Can you work these out from the model? Positions are in its coordinate system, mm. Coordinates: 2 decimals unless noted, no trailing zeros. Order: outer loops, then holes, each group sorted by start corner. A loop starts at its lowest first (then second) coordinate and runs counter-clockwise, first axis right, second up. Notation, with made-up numbers: (41, 46) - (73, 46) arc R13 cw to (73, 65) - close; hole circle Ø5 at (44, 22.25). An arc over 180 degrees is marked (long way). Return JSON: item names as keys, results as strings. Group by question number.
1) For pin 1 Ø0.8 at (y, z) = (-25.5, 1.5) entering from +X; pin 2 Ø1.2 at (y, z) = (97.5, 1.5) entering from -X; pin 3 Ø1.2 at (x, z) = (-18, 1) entering from -Y, each with a flat end and sliding along its axis, tell me the tip position at first contact or that it passes through.
2) Imagine slicing it at A-A (y = 120). Write out the boundary of the cut face in (x, z).
3) Imagine slicing it at D-D (x = -31.9). Write out the boundary of the cut face in (y, z), and give its area (3 significant figures).
4) If I drill on line 1 along Y through (x, z) = (-12.4, 1.3); line 2 along Y through (x, z) = (44, 1.05); line 3 along Y through (x, z) = (11, 1.35), over which ranges is the centre line in solid material (lowest first)?
5) Imagine slicing it at C-C (x = 2). Write out the boundary of the cut face in (y, z).
6) Imagine slicing it at B-B (x = -12.4). Write out the boundary of the cut face in (y, z).
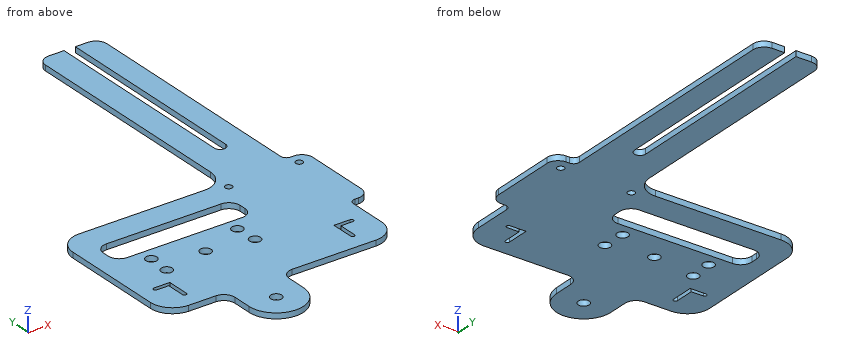
```python
from build123d import *

# Parameters (mm, degrees)
SKETCH1_W           = 200
SKETCH1_H           = 300
SKETCH1_W_2         = 96.214780988
SKETCH1_H_2         = 20
BOSS_EXTRUDE1_DEPTH = 2.5
SKETCH2_R           = 2.5
CUT_EXTRUDE1_DEPTH  = 10
CUT_EXTRUDE3_DEPTH  = 10
CUT_EXTRUDE4_REACH  = 182.936
SKETCH5_W           = 62
SKETCH5_H           = 13
FILLET2_R           = 5
FILLET3_R           = 10
FILLET4_R           = 5
CUT_EXTRUDE6_REACH  = 182.936
SKETCH7_R           = 1.6
FILLET5_R           = 2.5
CUT_EXTRUDE7_REACH  = 182.936
SKETCH8_R           = 2.5


with BuildPart() as part:
    # Sketch1 → Boss-Extrude1 (new body)
    with BuildSketch(Plane.XY):
        Rectangle(SKETCH1_W, SKETCH1_H)
        with Locations((51.892609506, 160)):
            Rectangle(SKETCH1_W_2, SKETCH1_H_2)
    extrude(amount=BOSS_EXTRUDE1_DEPTH)

    # Sketch2 → Cut-Extrude1 (cut)
    with BuildSketch(Plane.XY.offset(2.5)):
        with Locations((-12.4, -28.75)):
            Circle(SKETCH2_R)
        with Locations((7.6, 11.65)):
            Circle(SKETCH2_R)
        with Locations((-32.4, 11.65)):
            Circle(SKETCH2_R)
        Polygon((-44.5, 1.45), (-44.5, 3.25), (-37.2, 3.25), (-37.2, -7.05), (-39, -7.05), (-39, 1.45), align=None)
        Polygon((39, 1.45), (44.5, 1.45), (44.5, 3.25), (37.2, 3.25), (37.2, -7.05), (39, -7.05), align=None)
        with BuildLine():
            Line((-44.5, 1.45), (-44.5, 3.25))
            ThreePointArc((-44.5, 3.25), (-45.4, 2.35), (-44.5, 1.45))
        make_face()
        with BuildLine():
            ThreePointArc((-37.2, -7.05), (-38.1, -7.95), (-39, -7.05))
            Line((-39, -7.05), (-37.2, -7.05))
        make_face()
        with BuildLine():
            ThreePointArc((39, -7.05), (38.1, -7.95), (37.2, -7.05))
            Line((37.2, -7.05), (39, -7.05))
        make_face()
        with BuildLine():
            ThreePointArc((44.5, 3.25), (45.4, 2.35), (44.5, 1.45))
            Line((44.5, 1.45), (44.5, 3.25))
        make_face()
    extrude(amount=-CUT_EXTRUDE1_DEPTH, mode=Mode.SUBTRACT)

    # Sketch4 → Cut-Extrude3 (cut)
    with BuildSketch(Plane.XY.offset(2.5)):
        with BuildLine():
            Line((42.1, 170), (37, 170))
            Line((37, 170), (37, 77))
            ThreePointArc((37, 77), (39.55, 74.45), (42.1, 77))
            Line((42.1, 77), (42.1, 170))
        make_face()
        with BuildLine():
            Line((25, 53), (25, 170))
            Line((25, 170), (3.785219012, 170))
            Line((3.785219012, 170), (3.785219012, 150))
            Line((3.785219012, 150), (-100, 150))
            Line((-100, 150), (-100, -150))
            Line((-100, -150), (100, -150))
            Line((100, -150), (100, 170))
            Line((100, 170), (52.8, 170))
            Line((52.8, 170), (52.8, 55))
            Line((52.8, 55), (61.9, 55))
            Line((61.9, 55), (61.9, 15))
            Line((61.9, 15), (52.8, 15))
            Line((52.8, 15), (52.8, -15))
            Line((52.8, -15), (-0.095794877, -15))
            Line((-0.095794877, -15), (-0.095794877, -28.75))
            ThreePointArc((-0.095794877, -28.75), (-12.4, -41.054205123), (-24.704205123, -28.75))
            Line((-24.704205123, -28.75), (-24.704205123, -15))
            Line((-24.704205123, -15), (-52, -15))
            Line((-52, -15), (-52, 53))
            Line((-52, 53), (25, 53))
        make_face()
    extrude(amount=-CUT_EXTRUDE3_DEPTH, mode=Mode.SUBTRACT)

    # Sketch5 → Cut-Extrude4 (cut, up to next)
    with BuildSketch(Plane.XY.offset(2.5), mode=Mode.PRIVATE) as cut_extrude4_sk1:
        with Locations((-12.4, 34.409289568)):
            Rectangle(SKETCH5_W, SKETCH5_H)
    cut_extrude4_tool1 = extrude(cut_extrude4_sk1.sketch, amount=-CUT_EXTRUDE4_REACH, mode=Mode.PRIVATE) & part.part
    add(cut_extrude4_tool1.solids().sort_by_distance((-12.4, 34.40929, 2.5))[0], mode=Mode.SUBTRACT)

    # Fillet2
    fillet2_edges = [part.edges().sort_by_distance(p)[0] for p in [
        (-43.4, 40.909289568, 1.25),
        (18.6, 40.909289568, 1.25),
        (18.6, 27.909289568, 1.25),
        (-43.4, 27.909289568, 1.25),
    ]]
    fillet(fillet2_edges, radius=FILLET2_R)

    # Fillet3
    fillet3_edges = [part.edges().sort_by_distance(p)[0] for p in [
        (52.8, -15, 1.25),
        (25, 53, 1.25),
        (-52, 53, 1.25),
        (-52, -15, 1.25),
    ]]
    fillet(fillet3_edges, radius=FILLET3_R)

    # Fillet4
    fillet4_edges = [part.edges().sort_by_distance(p)[0] for p in [
        (-0.095794877, -15, 1.25),
        (61.9, 15, 1.25),
        (61.9, 55, 1.25),
        (-24.704205123, -15, 1.25),
        (25, 170, 1.25),
        (52.8, 170, 1.25),
    ]]
    fillet(fillet4_edges, radius=FILLET4_R)

    # Sketch7 → Cut-Extrude6 (cut, up to next)
    with BuildSketch(Plane.XY.offset(2.5), mode=Mode.PRIVATE) as cut_extrude6_sk1:
        with Locations((55.65, 49.91)):
            Circle(SKETCH7_R)
    cut_extrude6_tool1 = extrude(cut_extrude6_sk1.sketch, amount=-CUT_EXTRUDE6_REACH, mode=Mode.PRIVATE) & part.part
    # Sketch7 → Cut-Extrude6 (cut, up to next)
    with BuildSketch(Plane.XY.offset(2.5), mode=Mode.PRIVATE) as cut_extrude6_sk2:
        with Locations((23.65, 49.91)):
            Circle(SKETCH7_R)
    cut_extrude6_tool2 = extrude(cut_extrude6_sk2.sketch, amount=-CUT_EXTRUDE6_REACH, mode=Mode.PRIVATE) & part.part
    add(cut_extrude6_tool1.solids().sort_by_distance((55.65, 49.91, 2.5))[0], mode=Mode.SUBTRACT)
    add(cut_extrude6_tool2.solids().sort_by_distance((23.65, 49.91, 2.5))[0], mode=Mode.SUBTRACT)

    # Fillet5
    fillet5_edges = [part.edges().sort_by_distance(p)[0] for p in [
        (52.8, 15, 1.25),
        (52.8, 55, 1.25),
    ]]
    fillet(fillet5_edges, radius=FILLET5_R)

    # Sketch8 → Cut-Extrude7 (cut, up to next)
    with BuildSketch(Plane.XY.offset(2.5), mode=Mode.PRIVATE) as cut_extrude7_sk1:
        with Locations((7.1, 21.909289568)):
            Circle(SKETCH8_R)
    cut_extrude7_tool1 = extrude(cut_extrude7_sk1.sketch, amount=-CUT_EXTRUDE7_REACH, mode=Mode.PRIVATE) & part.part
    # Sketch8 → Cut-Extrude7 (cut, up to next)
    with BuildSketch(Plane.XY.offset(2.5), mode=Mode.PRIVATE) as cut_extrude7_sk2:
        with Locations((-31.9, 21.909289568)):
            Circle(SKETCH8_R)
    cut_extrude7_tool2 = extrude(cut_extrude7_sk2.sketch, amount=-CUT_EXTRUDE7_REACH, mode=Mode.PRIVATE) & part.part
    # Sketch8 → Cut-Extrude7 (cut, up to next)
    with BuildSketch(Plane.XY.offset(2.5), mode=Mode.PRIVATE) as cut_extrude7_sk3:
        with Locations((-12.4, 14.909289568)):
            Circle(SKETCH8_R)
    cut_extrude7_tool3 = extrude(cut_extrude7_sk3.sketch, amount=-CUT_EXTRUDE7_REACH, mode=Mode.PRIVATE) & part.part
    add(cut_extrude7_tool1.solids().sort_by_distance((7.1, 21.90929, 2.5))[0], mode=Mode.SUBTRACT)
    add(cut_extrude7_tool2.solids().sort_by_distance((-31.9, 21.90929, 2.5))[0], mode=Mode.SUBTRACT)
    add(cut_extrude7_tool3.solids().sort_by_distance((-12.4, 14.90929, 2.5))[0], mode=Mode.SUBTRACT)


solid = part.part
```
Calculated:
{
 "1": {"pin 1": "x = -0.1", "pin 2": "x = 25", "pin 3": "y = -39.99"},
 "2": {"outline": "(25, 0) - (37, 0) - (37, 2.5) - (25, 2.5) - close; (42.1, 0) - (52.8, 0) - (52.8, 2.5) - (42.1, 2.5) - close"},
 "3": {"outline": "(-15, 0) - (9.2, 0) - (9.2, 2.5) - (-15, 2.5) - close; (14.1, 0) - (19.41, 0) - (19.41, 2.5) - (14.1, 2.5) - close; (24.41, 0) - (27.91, 0) - (27.91, 2.5) - (24.41, 2.5) - close; (40.91, 0) - (53, 0) - (53, 2.5) - (40.91, 2.5) - close", "area": "113 mm2"},
 "4": {"line 1": "-41.05 to -31.25, -26.25 to 12.41, 17.41 to 27.91, 40.91 to 53", "line 2": "-14.93 to 1.45, 3.25 to 170", "line 3": "-15 to 27.91, 40.91 to 53"},
 "5": {"outline": "(-15.93, 0) - (27.91, 0) - (27.91, 2.5) - (-15.93, 2.5) - close; (40.91, 0) - (53, 0) - (53, 2.5) - (40.91, 2.5) - close"},
 "6": {"outline": "(-41.05, 0) - (-31.25, 0) - (-31.25, 2.5) - (-41.05, 2.5) - close; (-26.25, 0) - (12.41, 0) - (12.41, 2.5) - (-26.25, 2.5) - close; (17.41, 0) - (27.91, 0) - (27.91, 2.5) - (17.41, 2.5) - close; (40.91, 0) - (53, 0) - (53, 2.5) - (40.91, 2.5) - close"}
}
